Here's how the part is built. I have some questions about the finished solid (model axes, mm). Give positions to 0.01 mm unless a question says otherwise; leave off trailing zeros. Write each loop counter-clockwise with the first axis right and the second up, starting at its lowest first coordinate (ties: lowest second). Pieces come first, ordered by that corner, then holes. Notation, with made-up numbers: (49, 88.25) -> (60, 88.25) arc R7 cw to (60, 100.25) -> close; hole circle Ø7 at (-23, 53.5). An arc over 180 degrees is marked (long way). Return JSON: item names as keys, results as strings.
from build123d import *

# Parameters (mm, degrees)
SKETCH1_R           = 2.65
SKETCH1_R_2         = 2.55
SKETCH1_R_3         = 4.5
SKETCH1_W           = 25
SKETCH1_H           = 5
BOSS_EXTRUDE1_DEPTH = 5


with BuildPart() as part:
    # Sketch1 → Boss-Extrude1 (new body)
    with BuildSketch(Plane(origin=(0, 0, 0), x_dir=(1, 0, 0), z_dir=(0, 1, 0))):
        Polygon((0, 0), (0, 40), (0, 65), (-368.537, 65), (-368.537, -65), (0, -65), align=None)
        with Locations(Location((-12, 42.5, 0), (0, 0, 270))):
            Circle(SKETCH1_R, mode=Mode.SUBTRACT)
        with Locations(Location((-24.537, 33.5, 0), (0, 0, 270))):
            Circle(SKETCH1_R_2, mode=Mode.SUBTRACT)
        with Locations(Location((-24.537, -2.5, 0), (0, 0, 270))):
            Circle(SKETCH1_R_2, mode=Mode.SUBTRACT)
        with Locations(Location((-24.537, 15.5, 0), (0, 0, 270))):
            Circle(SKETCH1_R_3, mode=Mode.SUBTRACT)
        with Locations(Location((-12, -11.5, 0), (0, 0, 90))):
            Circle(SKETCH1_R, mode=Mode.SUBTRACT)
        with Locations(Location((-334.037, -51, 0), (0, 0, 270))):
            Circle(SKETCH1_R, mode=Mode.SUBTRACT)
        with Locations(Location((-234.037, -51, 0), (0, 0, 270))):
            Circle(SKETCH1_R, mode=Mode.SUBTRACT)
        with Locations(Location((-134.037, -51, 0), (0, 0, 270))):
            Circle(SKETCH1_R, mode=Mode.SUBTRACT)
        with Locations(Location((-34.037, -51, 0), (0, 0, 270))):
            Circle(SKETCH1_R, mode=Mode.SUBTRACT)
        with Locations(Location((-52, -11.5, 0), (0, 0, 270))):
            Circle(SKETCH1_R, mode=Mode.SUBTRACT)
        with Locations(Location((-52, 42.5, 0), (0, 0, 90))):
            Circle(SKETCH1_R, mode=Mode.SUBTRACT)
        with BuildLine():
            Line((-358.537, 20), (-344.537, 20))
            ThreePointArc((-344.537, 20), (-340.037, 15.5), (-344.537, 11))
            Line((-344.537, 11), (-358.537, 11))
            ThreePointArc((-358.537, 11), (-363.037, 15.5), (-358.537, 20))
        make_face(mode=Mode.SUBTRACT)
        with BuildLine():
            Line((-344.5, 0.05), (-358.5, 0.05))
            ThreePointArc((-358.5, 0.05), (-361.05, -2.5), (-358.5, -5.05))
            Line((-358.5, -5.05), (-344.5, -5.05))
            ThreePointArc((-344.5, -5.05), (-341.95, -2.5), (-344.5, 0.05))
        make_face(mode=Mode.SUBTRACT)
        with Locations((-297.055571099, 37)):
            Rectangle(SKETCH1_W, SKETCH1_H, mode=Mode.SUBTRACT)
        with Locations((-247.055571099, 37)):
            Rectangle(SKETCH1_W, SKETCH1_H, mode=Mode.SUBTRACT)
        with BuildLine():
            Line((-358.5, 36.05), (-344.5, 36.05))
            ThreePointArc((-344.5, 36.05), (-341.95, 33.5), (-344.5, 30.95))
            Line((-344.5, 30.95), (-358.5, 30.95))
            ThreePointArc((-358.5, 30.95), (-361.05, 33.5), (-358.5, 36.05))
        make_face(mode=Mode.SUBTRACT)
        with Locations((-197.055571099, 37)):
            Rectangle(SKETCH1_W, SKETCH1_H, mode=Mode.SUBTRACT)
        with Locations((-147.055571099, 37)):
            Rectangle(SKETCH1_W, SKETCH1_H, mode=Mode.SUBTRACT)
        with Locations((-97.055571099, 37)):
            Rectangle(SKETCH1_W, SKETCH1_H, mode=Mode.SUBTRACT)
    extrude(amount=BOSS_EXTRUDE1_DEPTH)


solid = part.part
1. If I drill on line 1 (X direction, y = 2.8, z = 11.5); line 2 (X direction, y = 3.5, z = 51); line 3 (Z direction, x = -24, y = 1.55), over which ranges is the centre line in solid material (lowest first)? Write a range as [from, to].
Taken from the geometry:
{"line 1": "x = [-368.54, -54.65], [-49.35, -14.65], [-9.35, 0]", "line 2": "x = [-368.54, -336.69], [-331.39, -236.69], [-231.39, -136.69], [-131.39, -36.69], [-31.39, 0]", "line 3": "z = [-65, -35.99], [-31.01, -19.97], [-11.03, 0.01], [4.99, 65]"}
2. Suppose I cut it at C-C, the plane y = 2. Count the separate pieces of the cut face and the enclosed holes in it, and give its area (3 significant figures).
Taken from the geometry:
{"separate pieces": "1", "enclosed holes": "19", "area": "46,600 mm²"}
3. Suppose I cut it at A-A, the plane z = -15.5. List the corners of the cut face in (x, y) for me.
Taken from the geometry:
{"outline": "(-368.54, 0) -> (-363.04, 0) -> (-363.04, 5) -> (-368.54, 5) -> close; (-340.04, 0) -> (-29.04, 0) -> (-29.04, 5) -> (-340.04, 5) -> close; (-20.04, 0) -> (0, 0) -> (0, 5) -> (-20.04, 5) -> close"}
4. If we mould it in two halves opening along Z, with no side actions, what happens to faces 1 (the face through (-21.5, 2.46, -18.82)), 2 (the face through (-187, 5, -1))? For each: released by +Z, released by -Z, zero draft, split by the parting line, or undercut.
Taken from the geometry:
{"face 1": "undercut", "face 2": "zero draft"}
5. Suppose I cut it at B-B, the plane x = -101.5. List the corners of the cut face in (y, z) for me, and give its area (3 significant figures).
Taken from the geometry:
{"outline": "(0, -65) -> (5, -65) -> (5, -39.5) -> (0, -39.5) -> close; (0, -34.5) -> (5, -34.5) -> (5, 65) -> (0, 65) -> close", "area": "625 mm²"}
6. For pin 1 Ø4.5 at (x, z) = (-24.537, 2.5) entering from -Y; pin 2 Ø2 at (x, z) = (-53, -34.5) entering from -Y, each with a flat end and sliding along its axis, tell me the tip position at first contact or that it passes through.
Taken from the geometry:
{"pin 1": "passes through", "pin 2": "stops at y = 0"}
